Autodesk Inventor part; units mm, degrees
ref_plane "YZ Plane" through (0, 0, 0) normal (1, 0, 0) x (0, 1, 0)
ref_plane "XZ Plane" through (0, 0, 0) normal (0, 1, 0) x (-1, 0, 0)
ref_plane "XY Plane" through (0, 0, 0) normal (0, 0, 1) x (1, 0, 0)
sketch "Sketch1" plane through (0, 0, 0) normal (0, 1, 0) x (-1, 0, 0)
  line L0 (-21, -21) -> (21, -21)
  line L1 (21, -21) -> (21, 21)
  line L2 (21, 21) -> (-21, 21)
  line L3 (-21, 21) -> (-21, -21)
  line L4 (-21, -21) -> (21, 21) construction
  line L5 (21, -21) -> (-21, 21) construction
  point P0 (0, 0)
  dimension "d0" = 42
  dimension "d1" = 42
extrude "Extrusion1" add sketch "Sketch1" along normal blind 9
chamfer "Chamfer1" distance 6 angle 45 4 edges at (21, 4.5, -21) (-21, 4.5, -21) (-21, 4.5, 21) (21, 4.5, 21)
sketch "Sketch2" plane through (0, 9, 0) normal (0, 1, 0) x (1, 0, 0)
  point P0 (0, 0)
sketch "Sketch3" plane through (0, 0, 0) normal (0, -1, 0) x (1, 0, 0)
  circle A0 centre (0, 0) radius 5
  dimension "d7" = 10
extrude "Extrusion2" cut sketch "Sketch3" against normal up to surface (9 mm away)
sketch "Sketch4" plane through (0, 9, 0) normal (0, 1, 0) x (1, 0, 0)
  circle A0 centre (-15.5, -15.5) radius 1.5
  line L0 (-15, -21) -> (15, -21)
  line L1 (-21, 15) -> (-21, -15)
  point P0 (0, 0)
  dimension "d10" = 3
  dimension "d11" = 5.5
  dimension "d12" = 5.5
extrude "Extrusion3" cut sketch "Sketch4" against normal up to surface (9 mm away)
mirror "Mirror1" about plane through (0, 0, 0) normal (1, 0, 0) of "Extrusion3"
mirror "Mirror2" about plane through (0, 0, 0) normal (0, 0, 1) of "Extrusion3", "Mirror1"
sketch "Sketch6" plane through (0, 0, 0) normal (0, -1, 0) x (1, 0, 0)
  circle A0 centre (15.5, -15.5) radius 1.5
  circle A1 centre (-15.5, -15.5) radius 1.5
  circle A2 centre (15.5, 15.5) radius 1.5
  circle A3 centre (-15.5, 15.5) radius 1.5
  circle A4 centre (0, 0) radius 5
  line L0 (15, 21) -> (21, 15)
  line L1 (-15, 21) -> (15, 21)
  line L2 (-21, 15) -> (-15, 21)
  line L3 (-21, -15) -> (-21, 15)
  line L4 (-15, -21) -> (-21, -15)
  line L5 (15, -21) -> (-15, -21)
  line L6 (21, -15) -> (15, -21)
  line L7 (21, 15) -> (21, -15)
  line L8 (8, -21) -> (-8, -21)
  line L9 (-8, -21) -> (-8, -25)
  line L10 (-8, -25) -> (8, -25)
  line L11 (8, -25) -> (8, -21)
  dimension "d20" = 16
  dimension "d21" = 8
  dimension "d24" = 4
extrude "Extrusion5" add sketch "Sketch6" against normal blind 4 contours L11 L10 L9 L5
fillet "Fillet1" radius 0.5 2 edges at (8, 2, -25) (-8, 2, -25)
sketch "Sketch7" plane through (15, 9, -21) normal (0, 0, -1) x (-1, 0, 0)
  line L0 (23, -5) -> (23, -9)
  line L1 (23, -9) -> (30, -9)
  line L2 (30, 0) -> (30, -9)
  line L3 (0, 0) -> (30, 0)
  line L4 (0, -9) -> (0, 0)
  line L5 (0, -9) -> (7, -9)
  line L6 (7, -9) -> (7, -5)
  line L7 (7, -5) -> (23, -5)
  line L8 (7, -5) -> (23, -5)
  line L9 (23, -5) -> (23, 0)
  line L10 (23, 0) -> (7, 0)
  line L11 (7, 0) -> (7, -5)
  point P0 (15, -9)
extrude "Extrusion6" cut sketch "Sketch7" against normal blind 10 contours L7 L11 L3 L9
sketch "Sketch8" plane through (15, 9, -11) normal (0, 0, -1) x (-1, 0, 0)
  line L0 (23, -5) -> (7, -5)
  line L1 (23, 0) -> (23, -5)
  line L2 (7, 0) -> (23, 0)
  line L3 (7, -5) -> (7, 0)
  line L4 (23, 0) -> (23, -5)
  line L5 (7, -4.3) -> (23, -4.3)
  line L6 (23, -4.3) -> (23, -4.8)
  line L7 (23, -4.8) -> (7, -4.8)
  line L8 (7, -4.8) -> (7, -4.3)
  point P0 (15, -9)
  dimension "d28" = 0.5
  dimension "d29" = 0.2
extrude "Extrusion7" add sketch "Sketch8" along normal blind 15 contours L7 L3 L5 L1
sketch "Sketch9" plane through (15, 9, -11) normal (0, 0, -1) x (-1, 0, 0)
  point P0 (15, -9)
sketch "Sketch10" plane through (0, 0, 0) normal (0, -1, 0) x (1, 0, 0)
  circle A0 centre (15.5, 15.5) radius 1.5
  circle A1 centre (15.5, 15.5) radius 3
  point P0 (0, 0)
  dimension "d32" = 6
extrude "Extrusion8" cut sketch "Sketch10" against normal blind 3
mirror "Mirror3" about plane through (0, 0, 0) normal (1, 0, 0) of "Extrusion8"
mirror "Mirror4" about plane through (0, 0, 0) normal (0, 0, 1) of "Extrusion8", "Mirror3"
sketch "Skizze11" plane through (0, 0, 0) normal (0, -1, 0) x (1, 0, 0)
  circle A0 centre (-15.5, -15.5) radius 3
  circle A1 centre (15.5, -15.5) radius 3
  circle A2 centre (-15.5, 15.5) radius 3
  circle A3 centre (15.5, 15.5) radius 3
  circle A4 centre (0, 0) radius 5
  arc A5 (-8, -24.5) -> (-7.5, -25) centre (-7.5, -24.5) ccw
  line L0 (-7.5, -25) -> (7.5, -25)
  arc A6 (7.5, -25) -> (8, -24.5) centre (7.5, -24.5) ccw
  line L1 (8, -24.5) -> (8, -21)
  line L2 (15, -21) -> (8, -21)
  line L3 (21, -15) -> (15, -21)
  line L4 (21, 15) -> (21, -15)
  line L5 (15, 21) -> (21, 15)
  line L6 (-15, 21) -> (15, 21)
  line L7 (-21, 15) -> (-15, 21)
  line L8 (-21, -15) -> (-21, 15)
  line L9 (-15, -21) -> (-21, -15)
  line L10 (-8, -21) -> (-15, -21)
  line L11 (-8, -21) -> (-8, -24.5)
extrude "Extrusion9" add sketch "Skizze11" along normal blind 9
equation "\"d12\" = d11"
Read the model definition and answer for the solid it produces. Units are mm, in the model's axes. A direction names the side the tool comes from. Round coordinates to 2 decimals unless told otherwise and drop trailing zeros. Loops run counter-clockwise (first coordinate to the right, second up) from the corner with the lowest first, then second, coordinate; pieces in that order, holes last. Notation, with made-up numbers: (-23, -36.5) - (30, -36.5) arc R22 cw to (30, -13.5) - close; hole circle Ø8 at (56, -30.5). An arc over 180 degrees is marked (long way). One line per question, with ' | ' between items. Start each with the question number.
Q1. Section B-B on z = 0 is taken. Give the vertices of the cut face in (x, y), plus the area to 3 significant figures.
Q2. Section D-D on x = -16 is taken. Give the vertices of the cut face in (y, z), plus the area to 3 significant figures.
Q3. Section A-A on y = -6.25 is taken. Give the vertices of the cut face in (x, z), plus the area to 3 significant figures.
Q4. For faces 4 (the cylindrical face through (13.1, -3.1, -17.3)), 5 (the flat face through (8, 7, -16)), 6 (the flat face through (-11, 0, -21)), 7 (the flat face through (8, -2, -23)), determine the directions among +Z, -Z, +X, -X, +Y, -Y from which every point of the face is accessible in a straight line to the end or side of a thin tool.
Q5. For a pull along X with two mould halves and no side action, classify faces 1 (the flat face through (0, -2, -25)), 2 (the cylindrical face through (-17, 6.04, 15.43)), 3 (the flat face through (18, 0, -18)) as +X half, -X half, draft (parallel to the pull), parting line (faces both ways), or undercut.
Q6. Section C-C on x = 0 is taken. Give the vertices of the cut face in (y, z).
Q7. Flat-ended cylindrical pins translate along their axes: pin 1 (1.8 mm diameter, centred on x = -15, z = 14.5, fed in from -Y); pin 2 (1.3 mm diameter, centred on x = 4, y = 7, fed in from -Z); pin 3 (0.6 mm diameter, centred on y = 4.5, z = -24, fed in from +X); pin 4 (12 mm diameter, centred on x = 3, z = -17.5, fed in from +Y). Find the tip coordinate at first contact, or state that the pin passes through.
Q8. Find the intervals of material crossed by L1, parallel to Z at x = -13.5, y = -5.75; L2, parallel to Z at x = 14, y = -2.5; L3, parallel to Y at x = -1.5, z = -13.5, in increasing order.
Established:
1) outline: (-21, -9) - (-5, -9) - (-5, 9) - (-21, 9) - close; (5, -9) - (21, -9) - (21, 9) - (5, 9) - close | area: 576 mm²
2) outline: (-9, -20) - (9, -20) - (9, -16.91) - (3, -16.91) - (3, -18.46) - (-9, -18.46) - close; (-9, -12.54) - (3, -12.54) - (3, -14.09) - (9, -14.09) - (9, 14.09) - (3, 14.09) - (3, 12.54) - (-9, 12.54) - close; (-9, 18.46) - (3, 18.46) - (3, 16.91) - (9, 16.91) - (9, 20) - (-9, 20) - close | area: 544 mm²
3) outline: (-21, -15) - (-15, -21) - (-8, -21) - (-8, -24.5) arc R0.5 ccw to (-7.5, -25) - (7.5, -25) arc R0.5 ccw to (8, -24.5) - (8, -21) - (15, -21) - (21, -15) - (21, 15) - (15, 21) - (-15, 21) - (-21, 15) - close; hole circle Ø6 at (-15.5, -15.5); hole circle Ø6 at (-15.5, 15.5); hole circle Ø10 at (0, 0); hole circle Ø6 at (15.5, -15.5); hole circle Ø6 at (15.5, 15.5) | area: 1,560 mm²
4) face 4: -Y | face 5: -Z, +Y | face 6: -Z, -X, +Y, -Y | face 7: -Z, +X, +Y, -Y
5) face 1: draft | face 2: undercut | face 3: +X half
6) outline: (-9, -25) - (4, -25) - (4, -11) - (4.2, -11) - (4.2, -26) - (4.7, -26) - (4.7, -11) - (9, -11) - (9, -5) - (-9, -5) - close; (-9, 5) - (9, 5) - (9, 21) - (-9, 21) - close
7) pin 1: y = 3 | pin 2: z = -11 | pin 3: x = 8 | pin 4: y = 9
8) L1: -21 to -17.74, -13.26 to 13.26, 17.74 to 21 | L2: -21 to -18.1, -12.9 to 12.9, 18.1 to 21 | L3: -9 to 4, 4.2 to 4.7
